Autodesk Fusion 360 part; units mm, degrees
sketch "Skizze1" plane through (0, 0, 0) normal (0, 0, 1) x (1, 0, 0)
  circle A0 centre (0, 0) radius 67.125
  dimension "d1" = 134.25
extrude "Extrusion1" add sketch "Skizze1" along normal blind 10
extrude "Extrusion2" add 1 faces at (20.1592, 3.4821, 10) along direction (0, 0, 1) blind 10
sketch "Skizze2" plane through (0, 0, 20) normal (0, 0, 1) x (-1, 0, 0)
  circle A0 centre (0, 0) radius 67.125
  line L0 (0, 0) -> (-60, 0)
  line L1 (-60, 0) -> (-60, -10)
  line L2 (-60, -10) -> (0, -10)
  line L3 (0, -10) -> (0, 0)
  line L4 (-60, 0) -> (0, 0)
  line L5 (0, 0) -> (0, 10)
  line L6 (0, 10) -> (-60, 10)
  line L7 (-60, 10) -> (-60, 0)
  line L8 (0, -10) -> (60, -10)
  line L9 (60, -10) -> (60, 10)
  line L10 (60, 10) -> (0, 10)
  line L11 (0, 10) -> (0, -10)
extrude "Extrusion3" add sketch "Skizze2" along normal blind 190 contours L0 L1 L2 L3 L4 L11 | L3 L5 L8 L9 L10 L11 | L0 L4 L5 L6 L7 L11
sketch "Skizze3" plane through (0, 0, 210) normal (0, 0, 1) x (-1, 0, 0)
  circle A0 centre (45, 0) radius 8
  circle A1 centre (-45, 0) radius 8
  dimension "d8" = 16
  dimension "d9" = 16
extrude "Extrusion4" add 1 faces at (-20, -10, 83.3333) along direction (0, -1, 0) blind 5
extrude "Extrusion5" add 1 faces at (20, 10, 83.3333) along direction (0, 1, 0) blind 5
sketch "Skizze4" plane through (0, 0, 210) normal (0, 0, 1) x (-1, 0, 0)
  circle A0 centre (0, 0) radius 5.25
  line L0 (0, 0) -> (-8, 0)
  line L1 (-8, 0) -> (0, 0)
  line L2 (0, 0) -> (8, 0)
  line L3 (0, 0) -> (0, 8)
  line L4 (0, 8) -> (0, -8)
  circle A1 centre (0, -8) radius 2
  circle A2 centre (8, 0) radius 2
  circle A3 centre (0, 8) radius 2
  circle A4 centre (-8, 0) radius 2
  line L5 (45, 0) -> (45, -12)
  line L6 (45, 0) -> (45, 12)
  line L7 (45, 12) -> (45, 0)
  line L8 (45, 0) -> (33, 0)
  line L9 (45, 0) -> (57, 0)
  line L10 (-45, 0) -> (-33, 0)
  line L11 (-33, 0) -> (-57, 0)
  line L12 (-45, 0) -> (-45, -12)
  line L13 (-45, -12) -> (-45, 12)
  circle A5 centre (-45, 0) radius 22.2036
  circle A6 centre (45, 0) radius 22.0227
  circle A7 centre (0, 0) radius 15
  circle A8 centre (-45, 12) radius 2
  circle A9 centre (-33, 0) radius 2
  circle A10 centre (-45, -12) radius 2
  circle A11 centre (-57, 0) radius 2
  circle A12 centre (45, -12) radius 2
  circle A13 centre (57, 0) radius 2
  circle A14 centre (45, 12) radius 2
  circle A15 centre (33, 0) radius 2
  dimension "d14" = 10.5
  dimension "d15" = 4
  dimension "d16" = 4
  dimension "d17" = 4
  dimension "d18" = 4
  dimension "d19" = 30
  dimension "d20" = 4
  dimension "d21" = 4
  dimension "d22" = 4
  dimension "d23" = 4
  dimension "d24" = 4
  dimension "d25" = 4
  dimension "d26" = 4
  dimension "d27" = 4
extrude "Extrusion6" cut 1 faces at (-20, -15, 83.3333) along direction (0, 1, 0) blind 30
extrude "Extrusion7" add sketch "Skizze4" sketch "Skizze3" against normal blind 190 of sketch 2 contours A0
sketch "Skizze5" plane through (0, 0, 210) normal (0, 0, 1) x (-1, 0, 0)
  circle A0 centre (45, 12) radius 2
  circle A1 centre (57, 0) radius 2
  circle A2 centre (45, -12) radius 2
  circle A3 centre (33, 0) radius 2
  circle A4 centre (45, 0) radius 22.0227
  circle A5 centre (45, 0) radius 8
  circle A6 centre (-45, 0) radius 8
  dimension "d32" = 16
  dimension "d33" = 16
extrude "Extrusion8" cut sketch "Skizze5" against normal blind 190 contours A5 | A6
extrude "Extrusion9" add 12 faces at (31.4364, 0.1671, 20) (46.386, -12.2526, 20) (46.386, 11.7474, 20) (57.8076, 0.4919, 20) (-0.4157, 8.5212, 20) (7.5843, -0.7199, 20) (0.9542, -8.597, 20) (-8.613, 0.4534, 20) (-34.1479, -0.5528, 20) (-43.614, -12.2526, 20) (-56.1924, 0.4919, 20) (-43.614, 11.7474, 20) along direction (0, 0, 1) blind 180
extrude "Extrusion10" add 3 faces at (38.0561, -11.8714, 210) (-7.5649, 5.256, 210) (-51.9063, -11.8242, 210) along direction (0, 0, 1) blind 10
extrude "Extrusion11" add 12 faces at (-56.1924, 0.4919, 200) (-43.614, 11.7474, 200) (-34.1479, -0.5528, 200) (-43.614, -12.2526, 200) (-0.4157, 8.5212, 200) (7.5843, -0.7199, 200) (0.9542, -8.597, 200) (-8.613, 0.4534, 200) (57.8076, 0.4919, 200) (46.386, 11.7474, 200) (31.4364, 0.1671, 200) (46.386, -12.2526, 200) along direction (0, 0, 1) blind 5
sketch "Skizze6" plane through (0, 0, 220) normal (0, 0, 1) x (-1, 0, 0)
  circle A0 centre (-45, 0) radius 8
  circle A1 centre (-33, 0) radius 2
  circle A2 centre (-57, 0) radius 2
  circle A3 centre (-45, -12) radius 2
  circle A4 centre (-45, 12) radius 2
  circle A5 centre (-45, 0) radius 22.2036
  circle A6 centre (45, 0) radius 20
  circle A7 centre (-45, 0) radius 20
  circle A8 centre (45, 0) radius 22.1359
  dimension "d42" = 40
  dimension "d43" = 40
extrude "Extrusion12" cut sketch "Skizze6" against normal blind 200 contours A5 | A8
sketch "Skizze7" plane through (0, 0, 0) normal (0, 0, -1) x (1, 0, 0)
  circle A0 centre (0, 0) radius 67.125
sketch "Skizze8" plane through (0, 0, 20) normal (0, 0, 1) x (-1, 0, 0)
  circle A0 centre (-45, 0) radius 20
  circle A1 centre (45, 0) radius 20
  circle A2 centre (0, 0) radius 67.125
  circle A3 centre (0, 0) radius 15
  line L0 (45, 20) -> (-45, 20)
  line L1 (-45, -20) -> (45, -20)
extrude "Extrusion13" add sketch "Skizze8" along normal up to surface (200 mm away) contours A0 A1 L0 L1
Read the model definition and answer for the solid it produces. Units are mm, in the model's axes. A direction names the side the tool comes from. Coordinates: 2 decimals unless noted, no trailing zeros. Loops run counter-clockwise (first coordinate to the right, second up) from the corner with the lowest first, then second, coordinate; pieces in that order, holes last.
(1) The part is cut by section A-A (z = 134). Determine the outline of the cut face in (x, y), and give its area (3 significant figures).
Solution:
outline: (-45, -20) - (45, -20) arc R20 ccw to (45, 20) - (-45, 20) arc R20 ccw to start; hole circle Ø16 at (-45, 0); hole circle Ø10.5 at (0, 0); hole circle Ø16 at (45, 0)
area: 4,370 mm2
(2) The part is cut by section B-B (y = 31). Determine the outline of the cut face in (x, z).
Solution:
outline: (-59.54, 0) - (59.54, 0) - (59.54, 20) - (-59.54, 20) - close
(3) The mould has two halves that part along Y. Classify faces 1 (the face through (-45, 0, 20)), 2 (the face through (65, 0, 121)), 3 (the face through (-1, 1, 0)): released by +Y, released by -Y, zero draft, split by the parting line, or undercut.
Solution:
face 1: undercut
face 2: split by the parting line
face 3: zero draft
(4) The part is cut by section C-C (y = -28.5). Determine the outline of the cut face in (x, z), and give its area (3 significant figures).
Solution:
outline: (-60.77, 0) - (60.77, 0) - (60.77, 20) - (-60.77, 20) - close
area: 2,430 mm2
(5) A tool of negligible diameter and unlimited length cuts with its end or side. For faces 4 (the face through (1, 20, 119)), 5 (the face through (-1, -20, 119)), 6 (the face through (-65, 0, 121)), 7 (the face through (-5, 1.6, 118.6)), from which of +Z, -Z, +X, -X, +Y, -Y can it reach the whole face along a straight path? Write none if from no direction.
Solution:
face 4: +Z, +X, -X, +Y
face 5: +Z, +X, -X, -Y
face 6: +Z, -X
face 7: +Z
(6) Consider line 1 along Y through (x, z) = (0, 213); line 2 along Y through (x, z) = (-33, 208.75); line 3 along X through (y, z) = (5.5, 110.5). Determine where each line is inside the solid, lowest interval first.
Solution:
line 1: y = -20 to -10, -6 to -5.25, 5.25 to 6, 10 to 20
line 2: y = -20 to -2, 2 to 20
line 3: x = -64.23 to -50.81, -39.19 to 39.19, 50.81 to 64.23
(7) Flat-ended cylindrical pins translate along their axes: pin 1 Ø1.2 at (x, y) = (0, -7.5) entering from +Z; pin 2 Ø1 at (y, z) = (18, 115.5) entering from +X; pin 3 Ø6 at (x, y) = (-48, 48.5) entering from +Z. Find the tip coordinate at first contact, or state that the pin passes through.
Solution:
pin 1: stops at z = 205
pin 2: stops at x = 54.68
pin 3: stops at z = 20
